```python
from build123d import *

# Parameters (mm, degrees)
BOSS_EXTRU_1_DEPTH      = 19
ESQUISSE2_W             = 18
ESQUISSE2_H             = 17
ENL_V_MAT_EXTRU_1_DEPTH = 12
TROU_TARAUD_M31_D       = 2.5
TROU_TARAUD_M31_DEPTH   = 8.5
TROU_TARAUD_M31_TIP     = 0.751075774
ESQUISSE7_W             = 25
ESQUISSE7_H             = 8.3
BOSS_EXTRU_2_DEPTH      = 7
CHANFREIN3_SIZE         = 3.25
TROU_TARAUD_M32_D       = 2.5
TROU_TARAUD_M32_DEPTH   = 6
TROU_TARAUD_M32_TIP     = 0.751075774


with BuildPart() as part:
    # Esquisse1 → Boss.-Extru.1 (new body)
    with BuildSketch(Plane(origin=(0, 0, 0), x_dir=(1, 0, 0), z_dir=(0, 1, 0))):
        with BuildLine():
            Line((-9.5, 20.7), (-9.5, 26.5))
            Line((-9.5, 26.5), (15.5, 26.5))
            Line((15.5, 26.5), (15.5, -26.5))
            Line((15.5, -26.5), (-9.5, -26.5))
            Line((-9.5, -26.5), (-9.5, -20.7))
            Line((-9.5, -20.7), (10, -20.7))
            ThreePointArc((10, -20.7), (10.848528137, -20.348528137), (11.2, -19.5))
            Line((11.2, -19.5), (11.2, 19.5))
            ThreePointArc((11.2, 19.5), (10.848528137, 20.348528137), (10, 20.7))
            Line((10, 20.7), (-9.5, 20.7))
        make_face()
    extrude(amount=BOSS_EXTRU_1_DEPTH)

    # Esquisse2 → Enlèv. mat.-Extru.1 (cut)
    with BuildSketch(Plane.XZ):
        with Locations((6.5, 18)):
            Rectangle(ESQUISSE2_W, ESQUISSE2_H)
        with Locations((6.5, -18)):
            Rectangle(ESQUISSE2_W, ESQUISSE2_H)
    extrude(amount=-ENL_V_MAT_EXTRU_1_DEPTH, mode=Mode.SUBTRACT)

    # Trou taraudé M31
    with Locations(Plane(origin=(0, 0, 0), x_dir=(-1, 0, 0), z_dir=(0, -1, 0))):
        with Locations((5.5, 23.6), (-13.35, 0), (5.5, -23.6)):
            Hole(TROU_TARAUD_M31_D / 2, depth=TROU_TARAUD_M31_DEPTH)
            with Locations((0, 0, -(TROU_TARAUD_M31_DEPTH + TROU_TARAUD_M31_TIP / 2))):  # 118° drill point
                Cone(0, TROU_TARAUD_M31_D / 2, TROU_TARAUD_M31_TIP, mode=Mode.SUBTRACT)

    # Esquisse7 → Boss.-Extru.2 (add)
    with BuildSketch(Plane(origin=(0, 19, 0), x_dir=(1, 0, 0), z_dir=(0, 1, 0))):
        with Locations((3, -24.85)):
            Rectangle(ESQUISSE7_W, ESQUISSE7_H)
        with Locations((3, 24.85)):
            Rectangle(ESQUISSE7_W, ESQUISSE7_H)
    extrude(amount=-BOSS_EXTRU_2_DEPTH)

    # Chanfrein3
    # the kernel refuses this chamfer: 3.25 mm, written as the material it adds along each edge
    with BuildSketch(Plane(origin=(11.2, 12, -9.5), x_dir=(0, 0.027495876610586424, -0.9996219169112968), z_dir=(1, 0, 0)), Plane(origin=(11.2, 12, 9.5), x_dir=(0, -0.9996219169112968, -0.027495876610586424), z_dir=(1, 0, 0))) as chanfrein3_piece_1:
        Polygon((CHANFREIN3_SIZE * 0.999621916911, -CHANFREIN3_SIZE * 0.0274958766106), (-CHANFREIN3_SIZE * 0.0274958766106, -CHANFREIN3_SIZE * 0.999621916911), (0, 0), align=None)
    extrude(amount=4.3)
    with BuildSketch(Plane(origin=(-9.5, 12, -26.5), x_dir=(0, -0.9996219169112968, 0.027495876610586424), z_dir=(1, 0, 0))) as chanfrein3_piece_2_section:
        Polygon((CHANFREIN3_SIZE * 0.999621916911, CHANFREIN3_SIZE * 0.0274958766106), (-CHANFREIN3_SIZE * 0.0274958766106, CHANFREIN3_SIZE * 0.999621916911), (0, 0), align=None)
    chanfrein3_piece_2 = extrude(amount=7, mode=Mode.PRIVATE)
    chanfrein3_piece_2 = split(chanfrein3_piece_2, bisect_by=Plane(origin=(-6, 10.864243408, -29), z_dir=(0, 0, 1)), keep=Keep.TOP, mode=Mode.PRIVATE)
    add(chanfrein3_piece_2)
    with BuildSketch(Plane(origin=(-2.5, 12, -26.5), x_dir=(-0.027495876610586424, -0.9996219169112968, 0), z_dir=(0, 0, 1)), Plane(origin=(-2.5, 12, 26.5), x_dir=(0.9996219169112966, 0.027495876610586428, 0), z_dir=(0, 0, -1))) as chanfrein3_piece_3:
        Polygon((CHANFREIN3_SIZE * 0.999621916911, CHANFREIN3_SIZE * 0.0274958766106), (-CHANFREIN3_SIZE * 0.0274958766106, CHANFREIN3_SIZE * 0.999621916911), (0, 0), align=None)
    extrude(amount=5.8)
    with BuildSketch(Plane(origin=(-9.5, 12, 26.5), x_dir=(0, 0.027495876610586424, 0.9996219169112968), z_dir=(1, 0, 0))) as chanfrein3_piece_4_section:
        Polygon((CHANFREIN3_SIZE * 0.999621916911, CHANFREIN3_SIZE * 0.0274958766106), (-CHANFREIN3_SIZE * 0.0274958766106, CHANFREIN3_SIZE * 0.999621916911), (0, 0), align=None)
    chanfrein3_piece_4 = extrude(amount=7, mode=Mode.PRIVATE)
    chanfrein3_piece_4 = split(chanfrein3_piece_4, bisect_by=Plane(origin=(-6, 10.864243408, 29), z_dir=(0, 0, -1)), keep=Keep.TOP, mode=Mode.PRIVATE)
    add(chanfrein3_piece_4)
    with BuildSketch(Plane(origin=(-9.5, 12, -26.5), x_dir=(0, -0.9996219169112968, 0.027495876610586424), z_dir=(1, 0, 0))) as chanfrein3_piece_5a_section:
        Polygon((CHANFREIN3_SIZE * 0.999621916911, CHANFREIN3_SIZE * 0.0274958766106), (-CHANFREIN3_SIZE * 0.0274958766106, CHANFREIN3_SIZE * 0.999621916911), (0, 0), align=None)
    chanfrein3_piece_5a = extrude(amount=15.357969711, mode=Mode.PRIVATE)
    chanfrein3_piece_5a = split(chanfrein3_piece_5a, bisect_by=Plane(origin=(-2.5, 10.864243408, -27.44984941), z_dir=(1, 0, 0)), keep=Keep.TOP, mode=Mode.PRIVATE)
    chanfrein3_piece_5a = split(chanfrein3_piece_5a, bisect_by=Plane(origin=(1.678984855, 10.864243408, -29), z_dir=(0, 0, 1)), keep=Keep.TOP, mode=Mode.PRIVATE)
    with BuildSketch(Plane(origin=(-2.5, 12, -34.857969711), x_dir=(-0.027495876610586424, -0.9996219169112968, 0), z_dir=(0, 0, 1))) as chanfrein3_piece_5b_section:
        Polygon((CHANFREIN3_SIZE * 0.999621916911, CHANFREIN3_SIZE * 0.0274958766106), (-CHANFREIN3_SIZE * 0.0274958766106, CHANFREIN3_SIZE * 0.999621916911), (0, 0), align=None)
    chanfrein3_piece_5b = extrude(amount=14.157969711, mode=Mode.PRIVATE)
    chanfrein3_piece_5b = split(chanfrein3_piece_5b, bisect_by=Plane(origin=(-1.428170713, 10.928170713, -26.5), z_dir=(0, 0, -1)), keep=Keep.TOP, mode=Mode.PRIVATE)
    chanfrein3_piece_5b = split(chanfrein3_piece_5b, bisect_by=Plane(origin=(-1.428170713, 10.928170713, -29), z_dir=(0, 0, 1)), keep=Keep.TOP, mode=Mode.PRIVATE)
    chanfrein3_piece_5 = chanfrein3_piece_5a & chanfrein3_piece_5b
    add(chanfrein3_piece_5)
    with BuildSketch(Plane(origin=(-9.5, 12, 26.5), x_dir=(0, 0.027495876610586424, 0.9996219169112968), z_dir=(1, 0, 0))) as chanfrein3_piece_6a_section:
        Polygon((CHANFREIN3_SIZE * 0.999621916911, CHANFREIN3_SIZE * 0.0274958766106), (-CHANFREIN3_SIZE * 0.0274958766106, CHANFREIN3_SIZE * 0.999621916911), (0, 0), align=None)
    chanfrein3_piece_6a = extrude(amount=15.357969711, mode=Mode.PRIVATE)
    chanfrein3_piece_6a = split(chanfrein3_piece_6a, bisect_by=Plane(origin=(1.678984855, 10.864243408, 29), z_dir=(0, 0, -1)), keep=Keep.TOP, mode=Mode.PRIVATE)
    chanfrein3_piece_6a = split(chanfrein3_piece_6a, bisect_by=Plane(origin=(-2.5, 10.864243408, 27.44984941), z_dir=(1, 0, 0)), keep=Keep.TOP, mode=Mode.PRIVATE)
    with BuildSketch(Plane(origin=(-2.5, 12, 34.857969711), x_dir=(0.9996219169112968, 0.027495876610586424, 0), z_dir=(0, 0, -1))) as chanfrein3_piece_6b_section:
        Polygon((CHANFREIN3_SIZE * 0.999621916911, CHANFREIN3_SIZE * 0.0274958766106), (-CHANFREIN3_SIZE * 0.0274958766106, CHANFREIN3_SIZE * 0.999621916911), (0, 0), align=None)
    chanfrein3_piece_6b = extrude(amount=14.157969711, mode=Mode.PRIVATE)
    chanfrein3_piece_6b = split(chanfrein3_piece_6b, bisect_by=Plane(origin=(-1.428170713, 10.928170713, 29), z_dir=(0, 0, -1)), keep=Keep.TOP, mode=Mode.PRIVATE)
    chanfrein3_piece_6b = split(chanfrein3_piece_6b, bisect_by=Plane(origin=(-1.428170713, 10.928170713, 26.5), z_dir=(0, 0, 1)), keep=Keep.TOP, mode=Mode.PRIVATE)
    chanfrein3_piece_6 = chanfrein3_piece_6a & chanfrein3_piece_6b
    add(chanfrein3_piece_6)
    # the kernel refuses this chamfer: 3.25 mm, written as the material it takes off along each edge
    with BuildSketch(Plane(origin=(15.5, 27.357969711, 29), x_dir=(0.027495876610586424, 0, -0.9996219169112968), z_dir=(0, -1, 0))) as chanfrein3_2_piece_1:
        Polygon((CHANFREIN3_SIZE * 0.999621916911, -CHANFREIN3_SIZE * 0.0274958766106), (-CHANFREIN3_SIZE * 0.0274958766106, -CHANFREIN3_SIZE * 0.999621916911), (0, 0), align=None)
    extrude(amount=23.715939422, mode=Mode.SUBTRACT)
    with BuildSketch(Plane(origin=(15.5, 27.357969711, -29), x_dir=(0.027495876610586424, 0, 0.9996219169112968), z_dir=(0, -1, 0))) as chanfrein3_2_piece_2:
        Polygon((CHANFREIN3_SIZE * 0.999621916911, CHANFREIN3_SIZE * 0.0274958766106), (-CHANFREIN3_SIZE * 0.0274958766106, CHANFREIN3_SIZE * 0.999621916911), (0, 0), align=None)
    extrude(amount=23.715939422, mode=Mode.SUBTRACT)

    # Trou taraudé M32
    with Locations(Plane(origin=(0, 19, 0), x_dir=(1, 0, 0), z_dir=(0, 1, 0))):
        with Locations((-4.15, 24.5), (-4.15, -24.5), (5.85, -24.5), (5.85, 24.5)):
            Hole(TROU_TARAUD_M32_D / 2, depth=TROU_TARAUD_M32_DEPTH)
            with Locations((0, 0, -(TROU_TARAUD_M32_DEPTH + TROU_TARAUD_M32_TIP / 2))):  # 118° drill point
                Cone(0, TROU_TARAUD_M32_D / 2, TROU_TARAUD_M32_TIP, mode=Mode.SUBTRACT)


solid = part.part
```
Can you work these out from the model? Positions are in its coordinate system, mm. A direction names the side the tool comes from. Coordinates: 2 decimals unless noted, no trailing zeros. Loops run counter-clockwise (first coordinate to the right, second up) from the corner with the lowest first, then second, coordinate; pieces in that order, holes last. Notation, with made-up numbers: (54, 48) - (59, 48) arc R15 cw to (59, 69) - close; hole circle Ø11 at (49.25, 0.5). An arc over 180 degrees is marked (long way). Use a Markdown table: item, result.
Item 1: For faces 4 (the face through (-2, 11, 20.7)), 5 (the face through (10, 12, -23)), 6 (the face through (-6.421, 4.31, 22.755)), which set-ups out of +Z, -Z, +X, -X, +Y, -Y let a thin tool reach every point of the face, with its end or its side?
Numbers:
| item | result |
|---|---|
| face 4 | -X, +Y, -Y |
| face 5 | -Z, +X, -Y |
| face 6 | -Y |
Item 2: I want a section at A-A on y = 3.5. Please give me the cut outline in (x, z), and give its area (3 significant figures).
Numbers:
| item | result |
|---|---|
| outline | (-9.5, -26.5) - (-2.5, -26.5) - (-2.5, -20.7) - (-9.5, -20.7) - close; (-9.5, 20.7) - (-2.5, 20.7) - (-2.5, 26.5) - (-9.5, 26.5) - close; (11.2, -9.5) - (15.5, -9.5) - (15.5, 9.5) - (11.2, 9.5) - close; hole circle Ø2.5 at (-5.5, -23.6); hole circle Ø2.5 at (-5.5, 23.6); hole circle Ø2.5 at (13.35, 0) |
| area | 148 mm2 |
Item 3: I want a section at C-C on y = 10. Please give me the cut outline in (x, z).
Numbers:
| item | result |
|---|---|
| outline | (-9.5, -27.75) - (-1.25, -27.75) - (-1.25, -20.7) - (-9.5, -20.7) - close; (-9.5, 20.7) - (-1.25, 20.7) - (-1.25, 27.75) - (-9.5, 27.75) - close; (11.2, -10.75) - (15.5, -10.75) - (15.5, 10.75) - (11.2, 10.75) - close |
Item 4: I want a section at B-B on x = 4. Please give me the cut outline in (y, z), and give its area (3 significant figures).
Numbers:
| item | result |
|---|---|
| outline | (12, -29) - (19, -29) - (19, -20.7) - (12, -20.7) - close; (12, 20.7) - (19, 20.7) - (19, 29) - (12, 29) - close |
| area | 116 mm2 |
Item 5: I want a section at D-D on z = 17.5. Please give me the cut outline in (x, y), and give its area (3 significant figures).
Numbers:
| item | result |
|---|---|
| outline | (11.2, 12) - (15.5, 12) - (15.5, 19) - (11.2, 19) - close |
| area | 30.1 mm2 |
Item 6: We'd pull the mould along X, two halves only. Please class faces 1 (the face through (-5.472, 9.121, 23.385)), 2 (the face through (2, 15, 29)), 3 (the face through (-2.5, 4, 24)): released by +X, released by -X, zero draft, split by the parting line, or undercut.
Numbers:
| item | result |
|---|---|
| face 1 | undercut |
| face 2 | zero draft |
| face 3 | released by +X |
Item 7: If I drill on probe 1 along X at (y, z) = (14.95, 24.5); probe 2 along Z at (x, y) = (-4.15, 17.1); probe 3 along Z at (x, y) = (-0.5, 12), over which ranges is the centre line in solid material (lowest first)? Write a range as from..to.
Numbers:
| item | result |
|---|---|
| probe 1 | x = -9.5..-5.4, -2.9..4.6, 7.1..15.5 |
| probe 2 | z = -29..-25.75, -23.25..-20.7, 20.7..23.25, 25.75..29 |
| probe 3 | z = -29..-20.7, 20.7..29 |
Item 8: Will these pins go through, and if not, where does the flat tip stop? pin 1 (1.7 mm diameter, centred on y = 6, z = 25, fed in from +X); pin 2 (2 mm diameter, centred on x = 5.85, z = -24.5, fed in from -Y); pin 3 (3 mm diameter, centred on y = 12, z = 17, fed in from -X).
Numbers:
| item | result |
|---|---|
| pin 1 | stops at x = -2.5 |
| pin 2 | stops at y = 12 |
| pin 3 | stops at x = 11.2 |
